Read the model definition and answer for the solid it produces. Units are mm, in the model's axes. Round coordinates to 2 decimals unless told otherwise and drop trailing zeros. Write each loop counter-clockwise with the first axis right and the second up, starting at its lowest first coordinate (ties: lowest second). Pieces come first, ordered by that corner, then holes. Notation, with made-up numbers: (-36, 46) - (-13, 46) arc R14 ccw to (-13, 58) - close; hole circle Ø4 at (54.25, -24.5). An arc over 180 degrees is marked (long way). One line per item, written item: value. Start each with the question number.
(1) Find the intervals of material crossed by L1, parallel to X at y = -1, z = -2.75; L2, parallel to Y at x = -1.25, z = -1; L3, parallel to Y at x = 0.5, z = -2.25, in increasing order.
(2) A cutting plane is placed at A-A, the plane y = 0. Determine the outline of the cut face in (x, z), plus the area to 3 significant figures.
(3) Flat-ended cylindrical pins translate along their axes: pin 1 Ø3 at (x, y) = (4, 0) entering from +Z; pin 2 Ø1 at (x, z) = (3, -4.5) entering from -Y; pin 3 Ø5.5 at (x, y) = (0, 0) entering from +Z; pin 4 Ø1.5 at (x, z) = (1.5, -5) entering from +Y. Find the tip coordinate at first contact, or state that the pin passes through.
(4) The mould has two halves that part along Y. Classify faces 1 (the face through (3.3, 5.6, -3.2)), 2 (the face through (0.74, -3.32, -3.29)), 3 (the face through (-6.5, 0, -3)), 4 (the face through (-3.3, -5.6, -3.2)): +Y half, -Y half, draft (parallel to the pull), parting line (faces both ways), or undercut.
(5) A cutting plane is placed at B-B, the plane z = -1. Determine the outline of the cut face in (x, y), plus the area to 3 significant figures.
from build123d import *

# Parameters (mm, degrees)
SKETCH2_R              = 8
CUT_EXTRUDE1_DEPTH     = 14.047988351
M8X1_25_TAPPED_HOLE1_D = 6.8
CHAMFER1_SIZE          = 0.5


with BuildPart() as part:
    # Sketch1 → Revolve1 (revolve)
    with BuildSketch(Plane(origin=(0, 0, 0), x_dir=(0, 0, -1), z_dir=(1, 0, 0)), mode=Mode.PRIVATE) as revolve1_sk:
        Polygon((0, 6.25), (1.010362971, 8), (5.489637029, 8), (6.5, 6.25), (6.5, 0), (0, 0), align=None)
    revolve(revolve1_sk.sketch.rotate(Axis((0, 0, 0), (0, 0, -1)), 90), axis=Axis((0, 0, 0), (0, 0, -1)))

    # Sketch2 → Cut-Extrude1 (cut, through all)
    with BuildSketch(Plane.XY):
        Circle(SKETCH2_R)
        Polygon((0, 7.505553499), (-6.5, 3.75277675), (-6.5, -3.75277675), (0, -7.505553499), (6.5, -3.75277675), (6.5, 3.75277675), align=None, mode=Mode.SUBTRACT)
    extrude(amount=-CUT_EXTRUDE1_DEPTH, mode=Mode.SUBTRACT)

    # M8x1.25 Tapped Hole1 (through all)
    with Locations(Plane.XY):
        with Locations((0, 0)):
            Hole(M8X1_25_TAPPED_HOLE1_D / 2)

    # Chamfer1
    chamfer1_edges = [part.edges().sort_by_distance(p)[0] for p in [
        (3.4, 0, 0),
        (3.4, 0, -6.5),
    ]]
    chamfer(chamfer1_edges, length=CHAMFER1_SIZE)


solid = part.part
Here are the results:
1. L1: -6.5 to -3.25, 3.25 to 6.5
1. L2: -6.78 to -3.16, 3.16 to 6.78
1. L3: -7.22 to -3.36, 3.36 to 7.22
2. outline: (-6.5, -6.36) - (-6.25, -6.5) - (-3.9, -6.5) - (-3.4, -6) - (-3.4, -0.5) - (-3.9, 0) - (-6.25, 0) - (-6.5, -0.14) - close; (3.4, -6) - (3.9, -6.5) - (6.25, -6.5) - (6.5, -6.36) - (6.5, -0.14) - (6.25, 0) - (3.9, 0) - (3.4, -0.5) - close
2. area: 39.7 mm²
3. pin 1: z = 0
3. pin 2: y = -6.06
3. pin 3: through
3. pin 4: y = 7.07
4. face 1: +Y half
4. face 2: undercut
4. face 3: draft
4. face 4: -Y half
5. outline: (-6.5, -3.75) - (0, -7.51) - (6.5, -3.75) - (6.5, 3.75) - (0, 7.51) - (-6.5, 3.75) - close; hole circle Ø6.8 at (0, 0)
5. area: 110 mm²
